Read the model definition and answer for the solid it produces. Units are mm, in the model's axes. Coordinates: 2 decimals unless noted, no trailing zeros. Loops run counter-clockwise (first coordinate to the right, second up) from the corner with the lowest first, then second, coordinate; pieces in that order, holes last. Notation, with made-up numbers: M -35,-7.5 L 12,-7.5 A8 ccw 12,-0.5 Z; hole C 5,-34.5 d1. An arc over 180 degrees is marked long. Put each result on its own line as item: value.
from build123d import *

# Parameters (mm, degrees)
BOSS_EXTRUDE1_DEPTH = 0.254
SKETCH2_R           = 4.699
CUT_EXTRUDE1_DEPTH  = 1.254
SKETCH3_W           = 2.54
SKETCH3_H           = 0.635
CUT_EXTRUDE2_DEPTH  = 1.254
CUT_EXTRUDE4_DEPTH  = 1.254
CUT_EXTRUDE5_DEPTH  = 1.254


with BuildPart() as part:
    # Sketch1 → Boss-Extrude1 (new body)
    with BuildSketch(Plane.XY):
        with BuildLine():
            Line((67.21146711, 76.191723231), (8.696654013, 17.676910134))
            Line((8.696654013, 17.676910134), (7.228954972, 14.133571205))
            ThreePointArc((7.228954972, 14.133571205), (14.666587579, 6.075099489), (15.105587123, -4.88230096))
            Line((15.105587123, -4.88230096), (18.648926052, -6.35))
            Line((18.648926052, -6.35), (101.401368334, -6.35))
            ThreePointArc((101.401368334, -6.35), (93.866160503, 38.880636728), (67.21146711, 76.191723231))
        make_face()
        with BuildLine():
            Line((88.672924278, 6.35), (27.86051193, 6.35))
            ThreePointArc((27.86051193, 6.35), (26.399857642, 10.93517908), (24.190484974, 15.210228852))
            Line((24.190484974, 15.210228852), (67.191354125, 58.211098004))
            ThreePointArc((67.191354125, 58.211098004), (82.13289044, 34.020557137), (88.672924278, 6.35))
        make_face(mode=Mode.SUBTRACT)
    extrude(amount=BOSS_EXTRUDE1_DEPTH)

    # Sketch2 → Cut-Extrude1 (cut, through all)
    with BuildSketch(Plane.XY.offset(0.254)):
        with Locations((22.225, 0)):
            Circle(SKETCH2_R)
        with Locations((36.195, 0)):
            Circle(SKETCH2_R)
        with Locations((61.722, 0)):
            Circle(SKETCH2_R)
        with Locations((75.692, 0)):
            Circle(SKETCH2_R)
        with Locations((95.25, 0)):
            Circle(SKETCH2_R)
        with Locations((15.715448212, 15.715448212)):
            Circle(SKETCH2_R)
        with Locations((25.593729945, 25.593729945)):
            Circle(SKETCH2_R)
        with Locations((43.644044748, 43.644044748)):
            Circle(SKETCH2_R)
        with Locations((53.522326482, 53.522326482)):
            Circle(SKETCH2_R)
        with Locations((92.004434954, 24.652514046)):
            Circle(SKETCH2_R)
        with Locations((82.48891971, 47.625)):
            Circle(SKETCH2_R)
        with Locations((67.351920908, 67.351920908)):
            Circle(SKETCH2_R)
    extrude(amount=-CUT_EXTRUDE1_DEPTH, mode=Mode.SUBTRACT)

    # Sketch3 → Cut-Extrude2 (cut, through all)
    with BuildSketch(Plane.XY.offset(0.254)):
        Polygon((15.266435406, 24.246691527), (17.06248663, 26.042742751), (17.511499436, 25.593729945), (15.715448212, 23.797678721), align=None)
        Polygon((44.991083167, 53.971339288), (43.195031942, 52.175288063), (43.644044748, 51.726275257), (45.440095973, 53.522326482), align=None)
        with Locations((29.21, -6.0325)):
            Rectangle(SKETCH3_W, SKETCH3_H)
        with Locations((68.707, -6.0325)):
            Rectangle(SKETCH3_W, SKETCH3_H)
        Polygon((29.230733674, 38.210989795), (31.026784898, 40.007041019), (31.475797704, 39.558028213), (29.67974648, 37.761976989), align=None)
        Polygon((56.845021246, 65.825277367), (55.048970022, 64.029226143), (55.497982828, 63.580213337), (57.294034052, 65.376264561), align=None)
        with Locations((48.9585, -6.0325)):
            Rectangle(SKETCH3_W, SKETCH3_H)
        with Locations((85.471, -6.0325)):
            Rectangle(SKETCH3_W, SKETCH3_H)
        Polygon((99.935462164, 14.437711971), (100.266998693, 11.919442024), (101.526133667, 12.085210288), (101.194597138, 14.603480236), align=None)
        Polygon((93.765504959, 37.464305742), (94.938831965, 37.950313702), (93.966816047, 40.296967714), (92.793489041, 39.810959755), align=None)
        Polygon((79.327792988, 62.471156422), (80.874047017, 60.456038938), (81.88160576, 61.229165953), (80.33535173, 63.244283437), align=None)
        Polygon((13.593916116, 7.005422516), (14.565932035, 4.658768503), (15.739259041, 5.144776462), (14.767243123, 7.491430475), align=None)
    extrude(amount=-CUT_EXTRUDE2_DEPTH, mode=Mode.SUBTRACT)

    # Sketch6 → Cut-Extrude4 (cut, through all)
    with BuildSketch(Plane.XY.offset(0.254)):
        with BuildLine():
            Line((22.27103518, 28.91642471), (40.321349984, 46.966739513))
            ThreePointArc((40.321349984, 46.966739513), (46.966739513, 46.966739513), (46.966739513, 40.321349984))
            Line((46.966739513, 40.321349984), (28.91642471, 22.27103518))
            ThreePointArc((28.91642471, 22.27103518), (22.27103518, 22.27103518), (22.27103518, 28.91642471))
        make_face()
        with BuildLine():
            Line((61.722, -4.699), (36.195, -4.699))
            ThreePointArc((36.195, -4.699), (31.496, 0), (36.195, 4.699))
            Line((36.195, 4.699), (61.722, 4.699))
            ThreePointArc((61.722, 4.699), (66.421, 0), (61.722, -4.699))
        make_face()
        with BuildLine():
            Line((95.25, -4.699), (75.692, -4.699))
            ThreePointArc((75.692, -4.699), (70.993, 0), (75.692, 4.699))
            Line((75.692, 4.699), (95.25, 4.699))
            ThreePointArc((95.25, 4.699), (99.949, 0), (95.25, -4.699))
        make_face()
        with BuildLine():
            ThreePointArc((26.924, 0), (24.874532533, 10.303368733), (19.038142977, 19.038142977))
            ThreePointArc((19.038142977, 19.038142977), (12.392753447, 19.038142977), (12.392753447, 12.392753447))
            ThreePointArc((12.392753447, 12.392753447), (16.191912687, 6.706909836), (17.526, 0))
            ThreePointArc((17.526, 0), (22.225, -4.699), (26.924, 0))
        make_face()
        with BuildLine():
            ThreePointArc((96.543320412, 25.868704739), (92.340835395, 38.248826381), (86.558373083, 49.9745))
            ThreePointArc((86.558373083, 49.9745), (80.13941971, 51.694453372), (78.419466338, 45.2755))
            ThreePointArc((78.419466338, 45.2755), (83.658215548, 34.652367484), (87.465549496, 23.436323353))
            ThreePointArc((87.465549496, 23.436323353), (93.220625647, 20.113628588), (96.543320412, 25.868704739))
        make_face()
    extrude(amount=-CUT_EXTRUDE4_DEPTH, mode=Mode.SUBTRACT)

    # Sketch5 → Cut-Extrude5 (cut, through all)
    with BuildSketch(Plane.XY.offset(0.254)):
        Polygon((55.857193073, 66.633500418), (68.493252435, 53.997441057), (81.501289898, 63.978859263), (67.351920908, 78.128228253), align=None)
    extrude(amount=-CUT_EXTRUDE5_DEPTH, mode=Mode.SUBTRACT)


solid = part.part
1) Find section B-B, the plane x = 74.5. Write down the section's boundary in (y, z).
Answer list:
outline: M -6.35,0 L -4.55,0 L -4.55,0.25 L -6.35,0.25 Z; M 4.55,0 L 6.35,0 L 6.35,0.25 L 4.55,0.25 Z; M 48.51,0 L 58.61,0 L 58.61,0.25 L 48.51,0.25 Z
2) Straight lines are drawn through the part: line 1 (X direction, y = 44, z = 0.2); line 2 (X direction, y = 1, z = 0.1); line 3 (Y direction, x = 33.5, z = 0.1). For each, find the intervals that lie inside material, in ascending order. Write a range as [from, to].
Answer list:
line 1: x = [35.02, 37.35], [48.33, 52.98], [77.25, 79.14], [89.74, 91.58]
line 2: x = [15.84, 17.5], [26.91, 31.6], [66.31, 71.1], [99.84, 101.6]
line 3: y = [-6.35, -3.85], [3.85, 6.35], [24.52, 26.85], [40.15, 42.48]
3) Given pin 1 Ø7.5 at (x, y) = (53.52, 53.52) entering from +Z, flat-ended and moving along its own axis, determine where the tip first touches the part or whether it passes through.
Answer list:
pin 1: passes through
4) Find section C-C, the plane y = 2. Write down the section's boundary in (x, z), plus the area to 3 significant figures.
Answer list:
outline: M 15.75,0 L 17.41,0 L 17.41,0.25 L 15.75,0.25 Z; M 26.85,0 L 31.94,0 L 31.94,0.25 L 26.85,0.25 Z; M 65.97,0 L 71.44,0 L 71.44,0.25 L 65.97,0.25 Z; M 99.5,0 L 101.58,0 L 101.58,0.25 L 99.5,0.25 Z
area: 3.63 mm^2
5) Find section A-A, the plane y = 30.5. Write down the section's boundary in (x, z), plus the area to 3 significant figures.
Answer list:
outline: M 21.52,0 L 23.85,0 L 23.85,0.25 L 21.52,0.25 Z; M 37.15,0 L 39.48,0 L 39.48,0.25 L 37.15,0.25 Z; M 83.5,0 L 85.26,0 L 85.26,0.25 L 83.5,0.25 Z; M 95.18,0 L 96.91,0 L 96.91,0.25 L 95.18,0.25 Z
area: 2.07 mm^2
